Source: CAD feature listing. Evaluate the final solid. Frame: model axes, mm. Round coordinates to 2 decimals unless told otherwise and drop trailing zeros. Loops run counter-clockwise (first coordinate to the right, second up) from the corner with the lowest first, then second, coordinate; pieces in that order, holes last.
(1) Section C-C, the plane x = -27. Return the cut outline in (y, z).
(2) Section A-A, the plane y = 0. Return the cut outline in (x, z).
(3) First-contact query: pin 1 Ø1.5 at (x, z) = (0, 2) entering from -Y; pin 2 Ø3 at (x, y) = (24.5, -18) entering from -Z; pin 3 Ø1.2 at (x, z) = (-26.5, 2.5) entering from +Y; pin 4 Ø2 at (y, z) = (-18, 2) entering from +X. Flat tips, straight axial feed; report the tip coordinate or a pass-through.
(4) Section B-B, the plane y = -18. Return the cut outline in (x, z).
(5) Material intervals for probe 1 along X at (y, z) = (-18, 2.7); probe 2 along X at (y, z) = (0, 2.9); probe 3 along Y at (x, z) = (24.5, 2.7), sorted ascending.
(6) Section D-D, the plane z = 2.4. Count the separate pieces of the cut face and the enclosed holes in it, plus the area to 3 significant figures.
Autodesk Fusion 360 part; units mm, degrees
sketch "スケッチ1" plane through (0, 0, 0) normal (0, 0, 1) x (1, 0, 0)
  line L0 (-20.5, 20) -> (20.5, 20)
  line L1 (20.5, 20) -> (20.5, 16)
  line L2 (20.5, 16) -> (28.7, 16)
  line L3 (28.7, 16) -> (28.7, 20)
  line L4 (28.7, 20) -> (35, 20)
  line L5 (35, 20) -> (35, -14)
  line L6 (35, -14) -> (29.5, -14)
  line L7 (29.5, -14) -> (29.5, -22)
  line L8 (29.5, -22) -> (19.5, -22)
  line L9 (19.5, -22) -> (19.5, -14)
  line L10 (19.5, -14) -> (-19.5, -14)
  line L11 (-19.5, -14) -> (-19.5, -22)
  line L12 (-19.5, -22) -> (-29.5, -22)
  line L13 (-29.5, -22) -> (-29.5, -14)
  line L14 (-29.5, -14) -> (-35, -14)
  line L15 (-35, -14) -> (-35, 20)
  line L16 (-35, 20) -> (-28.7, 20)
  line L17 (-28.7, 20) -> (-28.7, 16)
  line L18 (-28.7, 16) -> (-20.5, 16)
  line L19 (-20.5, 16) -> (-20.5, 20)
  line L20 (-22.5, 0) -> (22.5, 0)
  line L21 (-24.5, -22) -> (-24.5, -18)
  line L22 (24.5, -22) -> (24.5, -18)
  line L23 (-10, 16) -> (10, 16)
  line L24 (10, 16) -> (10, 20)
  line L25 (10, 20) -> (-10, 20)
  line L26 (-10, 20) -> (-10, 16)
  point P0 (0, 20)
  point P1 (0, -14)
  dimension "d1" = 16
  dimension "d2" = 4
  dimension "d4" = 14
  dimension "d5" = 8
  dimension "d6" = 41
  dimension "d7" = 8.2
  dimension "d8" = 8.2
  dimension "d9" = 70
  dimension "d10" = 45
  dimension "d16" = 39
  dimension "d17" = 10
  dimension "d18" = 10
  dimension "d19" = 4
  dimension "d24" = 20
  dimension "d25" = 4
extrude "押し出し1" add sketch "スケッチ1" along normal blind 4 contours L0 L1 L2 L3 L4 L5 L6 L7 L8 L9 L10 L11 L12 L13 L14 L15 L16 L17 L18 L19 L23 L24 L26
hole "穴1" at (-22.5, 0, 0) at (22.5, 0, 0) at (-24.5, -18, 0) at (24.5, -18, 0) direction (0, 0, 1) diameter 3.2 end through all
fillet "フィレット1" radius 1 12 edges at (35, 20, 2) (35, -14, 2) (29.5, -22, 2) (19.5, -22, 2) (-19.5, -22, 2) (-29.5, -22, 2) (-35, -14, 2) (-35, 20, 2) (10, 20, 2) (-10, 20, 2) (10, 16, 2) (-10, 16, 2)
fillet "フィレット2" radius 2 4 edges at (29.5, -14, 2) (19.5, -14, 2) (-19.5, -14, 2) (-29.5, -14, 2)
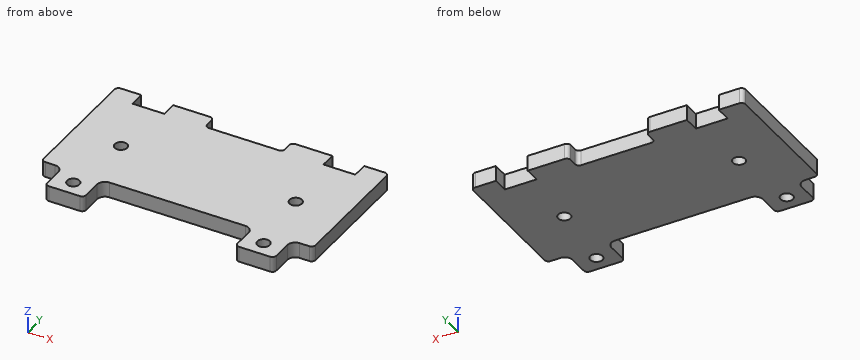
Output values:
1. outline: (-22, 0) - (16, 0) - (16, 4) - (-22, 4) - close
2. outline: (-35, 0) - (-24.1, 0) - (-24.1, 4) - (-35, 4) - close; (-20.9, 0) - (20.9, 0) - (20.9, 4) - (-20.9, 4) - close; (24.1, 0) - (35, 0) - (35, 4) - (24.1, 4) - close
3. pin 1: stops at y = -14
3. pin 2: passes through
3. pin 3: stops at y = 16
3. pin 4: stops at x = 29.5
4. outline: (-29.5, 0) - (-26.1, 0) - (-26.1, 4) - (-29.5, 4) - close; (-22.9, 0) - (-19.5, 0) - (-19.5, 4) - (-22.9, 4) - close; (19.5, 0) - (22.9, 0) - (22.9, 4) - (19.5, 4) - close; (26.1, 0) - (29.5, 0) - (29.5, 4) - (26.1, 4) - close
5. probe 1: x = -29.5 to -26.1, -22.9 to -19.5, 19.5 to 22.9, 26.1 to 29.5
5. probe 2: x = -35 to -24.1, -20.9 to 20.9, 24.1 to 35
5. probe 3: y = -22 to -19.6, -16.4 to 16
6. separate pieces: 1
6. enclosed holes: 4
6. area: 2,360 mm2
